Drawing for the job (mm, zero at the part's lowest x, y, z). A direction names the side the tool comes from. Give positions to 0.01 mm unless a question says otherwise; leave off trailing zeros. Loops run counter-clockwise (first coordinate to the right, second up) from the corner with the lowest first, then second, coordinate; pieces in that order, holes last.
1) Two-plate mould, pull along Y, no slides. Class the marked faces 3, 4, 5 and 6: +Y half, -Y half, draft (parallel to the pull), parting line (faces both ways), or undercut.
2) Band-saw the part on C-C on y = 36.5. List the corners of the cut face in (x, z), then the cut area to 3 significant figures.
3) 3-axis set-ups, long thin cutter, end or side, ignore diameter. For the marked faces 1 and 2: which of +Z, -Z, +X, -X, +Y, -Y reach the whole face in a straight line?
4) Flat gauge pin, fed straight in: P1, Ø10, axis at x = 52, y = 12, coming from the +Z side. Where does the tip first touch, or does it go through?
5) Band-saw the part on D-D on x = 69. List the corners of the cut face in (y, z) (1 decimal).
6) Band-saw the part on B-B on x = 28.5. List the corners of the cut face in (y, z) (1 decimal).
7) Band-saw the part on A-A on z = 9.5. List the corners of the cut face in (x, y) (1 decimal).
8) Wall check: line 1 (Y direction, x = 58.5, z = 8.5) (1 decimal); line 2 (X direction, y = 33.5, z = 9.75); line 3 (Z direction, x = 7.5, y = 29). Give the ranges that are in metal, low to high.
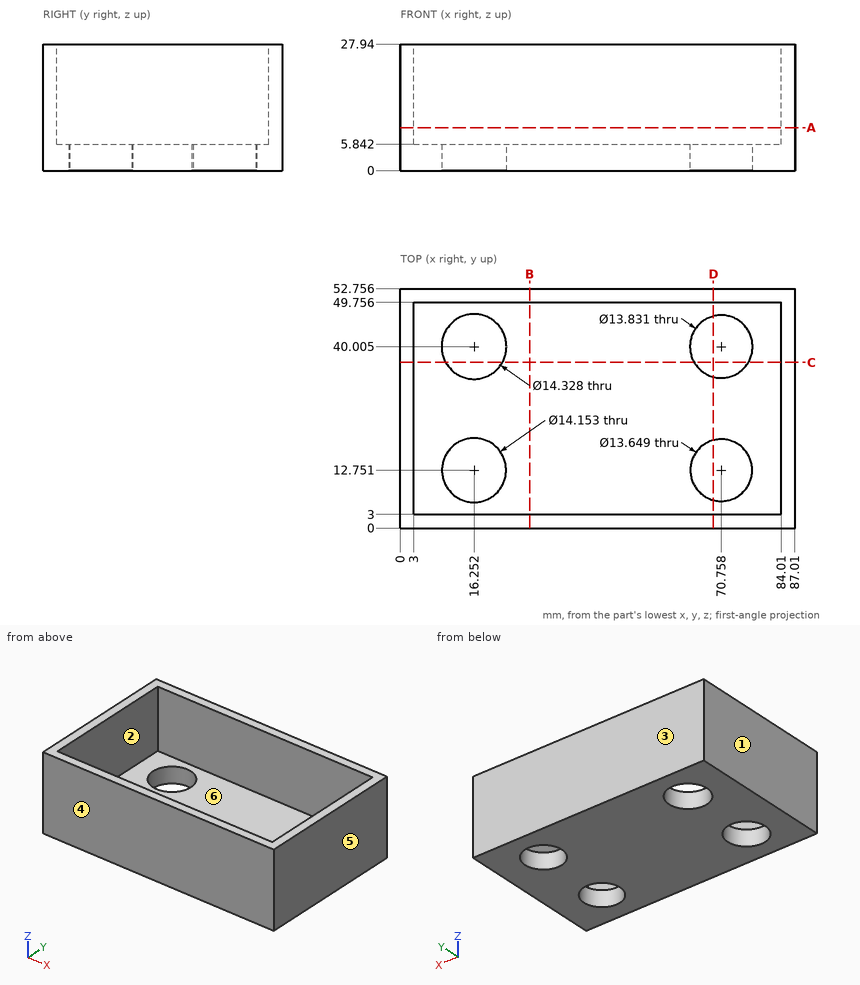
Findings below:
1. face 3: +Y half
1. face 4: -Y half
1. face 5: draft
1. face 6: undercut
2. outline: (0, 0) - (10, 0) - (10, 5.84) - (3, 5.84) - (3, 27.94) - (0, 27.94) - close; (22.5, 0) - (64.8, 0) - (64.8, 5.84) - (22.5, 5.84) - close; (76.72, 0) - (87.01, 0) - (87.01, 27.94) - (84.01, 27.94) - (84.01, 5.84) - (76.72, 5.84) - close
2. area: 498 mm2
3. face 1: +Z, -Z, -X, +Y, -Y
3. face 2: +Z
4. P1: stops at z = 5.84
5. outline: (0, 0) - (6.2, 0) - (6.2, 5.8) - (3, 5.8) - (3, 27.9) - (0, 27.9) - close; (19.3, 0) - (33.3, 0) - (33.3, 5.8) - (19.3, 5.8) - close; (46.7, 0) - (52.8, 0) - (52.8, 27.9) - (49.8, 27.9) - (49.8, 5.8) - (46.7, 5.8) - close
6. outline: (0, 0) - (52.8, 0) - (52.8, 27.9) - (49.8, 27.9) - (49.8, 5.8) - (3, 5.8) - (3, 27.9) - (0, 27.9) - close
7. outline: (0, 0) - (87, 0) - (87, 52.8) - (0, 52.8) - close; hole (3, 3) - (84, 3) - (84, 49.8) - (3, 49.8) - close
8. line 1: y = 0 to 3, 49.8 to 52.8
8. line 2: x = 0 to 3, 84.01 to 87.01
8. line 3: z = 0 to 5.84
